Design review of the part built by this model. Coordinates are the model's own, in mm. A direction names the side the tool comes from. Coordinates: 2 decimals unless noted, no trailing zeros. Loops run counter-clockwise (first coordinate to the right, second up) from the corner with the lowest first, then second, coordinate; pieces in that order, holes last. Notation, with made-up numbers: M -34.75,-4.75 L -28.75,-4.75 A24 cw -28.75,8.25 Z; hole C 22.25,-8.75 d1. An arc over 180 degrees is marked long. Put each result on its own line as item: value. Start each with the question number.
(1) The part is to be moulded in two halves that separate along Y. For faces 3 (the conical face through (52.872, 16.65, 7.485)), 4 (the flat face through (8.5, -17.5, 4.318)), 5 (the flat face through (-1, 12, -7.62)), say which applies: +Y half, -Y half, draft (parallel to the pull), parting line (faces both ways), or undercut.
(2) Take a section at B-B, the plane z = -1.25. Give the boundary of the cut face in (x, y) (1 decimal), then the cut area to 3 significant figures.
(3) For faces 1 (the flat face through (-25, -41, 13.97)), 2 (the flat face through (13, -56, -3.81)), list the 3-axis set-ups (+Z, -Z, +X, -X, +Y, -Y) from which the entire face can be reached by the end or side of a thin tool; tool diameter is ignored.
(4) For probe 1 along Y at (x, z) = (0, 11.5); probe 2 along Y at (x, z) = (0, 12.1); probe 3 along Y at (x, z) = (0, -2.5), list the stretches that pass through material, from the lowest coordinate up. Write a range as [from, to].
(5) Clearance check with a flat-ended pin moving along its axis: pin 1 (1.5 mm diameter, centred on x = 35.5, z = -2, fed in from +Y). State where the tip first meets the part, or that it passes through.
(6) Take a section at A-A, the plane z = 6.75. Give the boundary of the cut face in (x, y) (1 decimal), then the cut area to 3 significant figures.
```python
from build123d import *

# Parameters (mm, degrees)
SKETCH1_R                   = 58.42
BOSS_EXTRUDE1_DEPTH         = 13.97
SKETCH2_R                   = 46.99
SKETCH2_R_2                 = 12.7
CUT_EXTRUDE1_DEPTH          = 9.652
FILLET1_R                   = 6.35
SKETCH3_R                   = 60.96
BOSS_EXTRUDE2_DEPTH         = 7.62
SKETCH4_R                   = 7.9375
CUT_EXTRUDE2_DEPTH          = 89.872781548
SKETCH5_R                   = 60.96
SKETCH5_R_2                 = 58.42
FLANGEWIDTHMACHINED_DEPTH   = 3.81
SKETCH7_R                   = 58.42
SKETCH7_R_2                 = 55.5625
CUT_EXTRUDE5_DEPTH          = 17.78
SKETCH6_R                   = 60.96
SKETCH6_R_2                 = 59.8805
FLANGE_DEPTH_MACHINED_DEPTH = 89.024835132
DRAFT1_ANGLE                = 1
FILLET2_R                   = 0.8128
FILLET3_R                   = 1.905


with BuildPart() as part:
    # Sketch1 → Boss-Extrude1 (new body)
    with BuildSketch(Plane.XY):
        Circle(SKETCH1_R)
    extrude(amount=BOSS_EXTRUDE1_DEPTH)

    # Sketch2 → Cut-Extrude1 (cut)
    with BuildSketch(Plane.XY.offset(13.97)):
        Circle(SKETCH2_R)
        Circle(SKETCH2_R_2, mode=Mode.SUBTRACT)
    extrude(amount=-CUT_EXTRUDE1_DEPTH, mode=Mode.SUBTRACT)

    # Fillet1
    fillet1_edges = [part.edges().sort_by_distance(p)[0] for p in [
        (-46.99, 0, 4.318),
        (-12.7, 0, 4.318),
    ]]
    fillet(fillet1_edges, radius=FILLET1_R)

    # Sketch3 → Boss-Extrude2 (add)
    with BuildSketch(Plane(origin=(0, 0, 0), x_dir=(-1, 0, 0), z_dir=(0, 0, -1))):
        with Locations(Location((0, 0, 0), (0, 0, 180))):
            Circle(SKETCH3_R)
    extrude(amount=BOSS_EXTRUDE2_DEPTH)

    # Sketch4 → Cut-Extrude2 (cut, through all)
    with BuildSketch(Plane.XY.offset(13.97)):
        Circle(SKETCH4_R)
    extrude(amount=-CUT_EXTRUDE2_DEPTH, mode=Mode.SUBTRACT)

    # Sketch5 → FlangeWidthMachined (cut)
    with BuildSketch(Plane.XY):
        Circle(SKETCH5_R)
        Circle(SKETCH5_R_2, mode=Mode.SUBTRACT)
    extrude(amount=-FLANGEWIDTHMACHINED_DEPTH, mode=Mode.SUBTRACT)

    # Sketch7 → Cut-Extrude5 (cut)
    with BuildSketch(Plane.XY.offset(13.97)):
        Circle(SKETCH7_R)
        Circle(SKETCH7_R_2, mode=Mode.SUBTRACT)
    extrude(amount=-CUT_EXTRUDE5_DEPTH, mode=Mode.SUBTRACT)

    # Sketch6 → Flange Depth Machined (cut, through all)
    with BuildSketch(Plane.XY.offset(-3.81)):
        Circle(SKETCH6_R)
        Circle(SKETCH6_R_2, mode=Mode.SUBTRACT)
    extrude(amount=-FLANGE_DEPTH_MACHINED_DEPTH, mode=Mode.SUBTRACT)

    # Draft1
    draft1_faces = [part.faces().sort_by_distance(p)[0] for p in [
        (-55.5625, 0, 5.08),
    ]]
    draft(draft1_faces, Plane.XY, DRAFT1_ANGLE)

    # Fillet2
    fillet2_edges = [part.edges().sort_by_distance(p)[0] for p in [
        (-55.629003797, 0, -3.81),
    ]]
    fillet(fillet2_edges, radius=FILLET2_R)

    # Fillet3
    fillet3_edges = [part.edges().sort_by_distance(p)[0] for p in [
        (-59.8805, 0, -7.62),
        (-59.8805, 0, -3.81),
    ]]
    fillet(fillet3_edges, radius=FILLET3_R - 0.0001)  # a hair under: the kernel refuses the full size


solid = part.part
```
Computed values:
1. face 3: parting line
1. face 4: undercut
1. face 5: draft
2. outline: C 0,0 d111.2; hole C 0,0 d15.9
2. area: 9,510 mm^2
3. face 1: +Z, +X, -X, +Y, -Y
3. face 2: +Z
4. probe 1: y = [-55.36, -46.99], [-12.7, -7.94], [7.94, 12.7], [46.99, 55.36]
4. probe 2: y = [-55.35, -46.99], [-12.7, -7.94], [7.94, 12.7], [46.99, 55.35]
4. probe 3: y = [-55.61, -7.94], [7.94, 55.61]
5. pin 1: stops at y = 43.4
6. outline: C 0,0 d110.9; C 0,0 d28.1; hole C 0,0 d91.3; hole C 0,0 d15.9
6. area: 3,540 mm^2
